Read the model definition and answer for the solid it produces. Units are mm, in the model's axes. Face numbers are marked on the shaded views. A direction names the side the tool comes from. Coordinates: 2 decimals unless noted, no trailing zeros. Write each loop counter-clockwise with the first axis right and the second up, starting at its lowest first coordinate (ties: lowest second). Pieces come first, ordered by that corner, then holes. Notation, with made-up numbers: M -9.5,-22.75 L 24.5,-22.75 A15 cw 24.5,-1.75 Z; hole C -6,80.5 d3. An arc over 180 degrees is marked long. Write item = value, one per line.
from build123d import *

# Parameters (mm, degrees)
SKETCH_1_W          = 110
SKETCH_1_H          = 51
EXTRUDE_1_DEPTH     = 5
EXTRUDE_2_DEPTH     = 25
SKETCH_3_R          = 1.55
CUT_EXTRUDE_1_DEPTH = 123.613771256
EXTRUDE_3_DEPTH     = 35


with BuildPart() as part:
    # Sketch 1 → Extrude 1 (new body)
    with BuildSketch(Plane(origin=(0, 0, 0), x_dir=(1, 0, 0), z_dir=(0, 1, 0))):
        with Locations((12.685483871, -8.911290323)):
            Rectangle(SKETCH_1_W, SKETCH_1_H)
    extrude(amount=EXTRUDE_1_DEPTH)



with BuildPart() as body_2:
    # Sketch 2 → Extrude 2 (new body)
    with BuildSketch(Plane.XZ):
        Polygon((-42.314516129, 34.411290323), (-47.314516129, 34.411290323), (-47.314516129, -16.588709677), (-47.314516129, -21.588709677), (67.685483871, -21.588709677), (67.685483871, -16.588709677), (-42.314516129, -16.588709677), align=None)
    extrude(amount=-EXTRUDE_2_DEPTH)

    # Sketch 3 → Cut-Extrude 1 (cut, through all)
    with BuildSketch(Plane.ZY.offset(47.314516129)):
        with Locations((-9.775923567, 12.5)):
            Circle(SKETCH_3_R)
        with Locations((6.411290323, 12.5)):
            Circle(SKETCH_3_R)
        with Locations((22.411290323, 12.5)):
            Circle(SKETCH_3_R)
    extrude(amount=-CUT_EXTRUDE_1_DEPTH, mode=Mode.SUBTRACT)


with BuildPart() as part_1:
    add(part.part)

    add(body_2.part)  # Extrude 3 merges body 2
    # Sketch 4 → Extrude 3 (add)
    with BuildSketch(Plane.XZ):
        Polygon((67.685483871, 29.411290323), (67.685483871, 34.411290323), (62.685483871, 34.411290323), (16.301510032, 34.411290323), (16.301510032, 29.411290323), (62.685483871, 29.411290323), (62.685483871, -16.588709677), (67.685483871, -16.588709677), align=None)
    extrude(amount=EXTRUDE_3_DEPTH)


solid = part_1.part
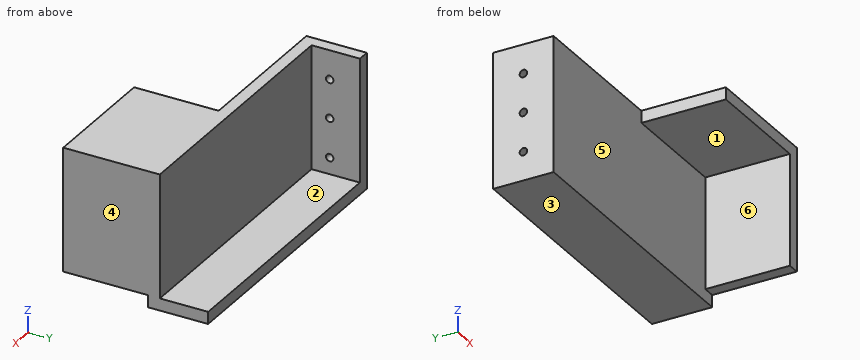
Item 1: Which of the six approach directions +Z, -Z, +X, -X, +Y, -Y give full straight-line access (tool end or side, diameter ignored) to the marked faces 1, 2 and 3?
Worked answers:
face_1 = -Z, -X, -Y
face_2 = +Z, +X, +Y
face_3 = -Z, +X, -X, +Y, -Y
Item 2: Find section C-C (x = 36). Determine the outline of the cut face in (y, z), and give its area (3 significant figures).
Worked answers:
outline = M -35,29.41 L 0,29.41 L 0,-21.59 L 25,-21.59 L 25,-16.59 L 5,-16.59 L 5,34.41 L -35,34.41 Z
area = 555 mm²
Item 3: Find section D-D (y = -19). Determine the outline of the cut face in (x, z), and give its area (3 significant figures).
Worked answers:
outline = M 16.3,29.41 L 62.69,29.41 L 62.69,-16.59 L 67.69,-16.59 L 67.69,34.41 L 16.3,34.41 Z
area = 487 mm²
Item 4: For a pull along X with two mould halves and no side action, classify the marked faces 4, 5 and 6 as released by +X, released by -X, zero draft, split by the parting line, or undercut.
Worked answers:
face_4 = released by +X
face_5 = zero draft
face_6 = released by -X
Item 5: Flat-ended cylindrical pins translate along their axes: pin 1 (5 mm diameter, centred on x = -23.5, z = 26.5, fed in from -Y); pin 2 (2.5 mm diameter, centred on y = 12.5, z = -9.78, fed in from +X); pin 3 (22 mm diameter, centred on y = 19.5, z = 13.5, fed in from +X); pin 4 (10 mm diameter, centred on x = 8.5, y = 18.5, fed in from +Z). Find the tip coordinate at first contact, or state that the pin passes through.
Worked answers:
pin_1 = 0
pin_2 = through
pin_3 = -42.31
pin_4 = -16.59
Item 6: Consider line 1 along Z through (x, y) = (-44, 12); line 2 along Y through (x, z) = (-8.5, -5.5); line 3 along Z through (x, y) = (-31, 11). Determine where each line is inside the solid, lowest interval first. Write a range as from..to.
Worked answers:
line_1 = -21.59..-11.24, -8.31..4.94, 7.88..20.94, 23.88..34.41
line_2 = 0..5
line_3 = -21.59..-16.59
Item 7: Find section A-A (y = 12.5). Determine the outline of the cut face in (x, z).
Worked answers:
outline = M -47.31,-21.59 L 67.69,-21.59 L 67.69,-16.59 L -42.31,-16.59 L -42.31,-11.33 L -47.31,-11.33 Z; M -47.31,-8.23 L -42.31,-8.23 L -42.31,4.86 L -47.31,4.86 Z; M -47.31,7.96 L -42.31,7.96 L -42.31,20.86 L -47.31,20.86 Z; M -47.31,23.96 L -42.31,23.96 L -42.31,34.41 L -47.31,34.41 Z
Item 8: Find section B-B (z = 12). Determine the outline of the cut face in (x, y), and give its area (3 significant figures).
Worked answers:
outline = M -47.31,0 L 62.69,0 L 62.69,-35 L 67.69,-35 L 67.69,5 L -42.31,5 L -42.31,25 L -47.31,25 Z
area = 850 mm²
